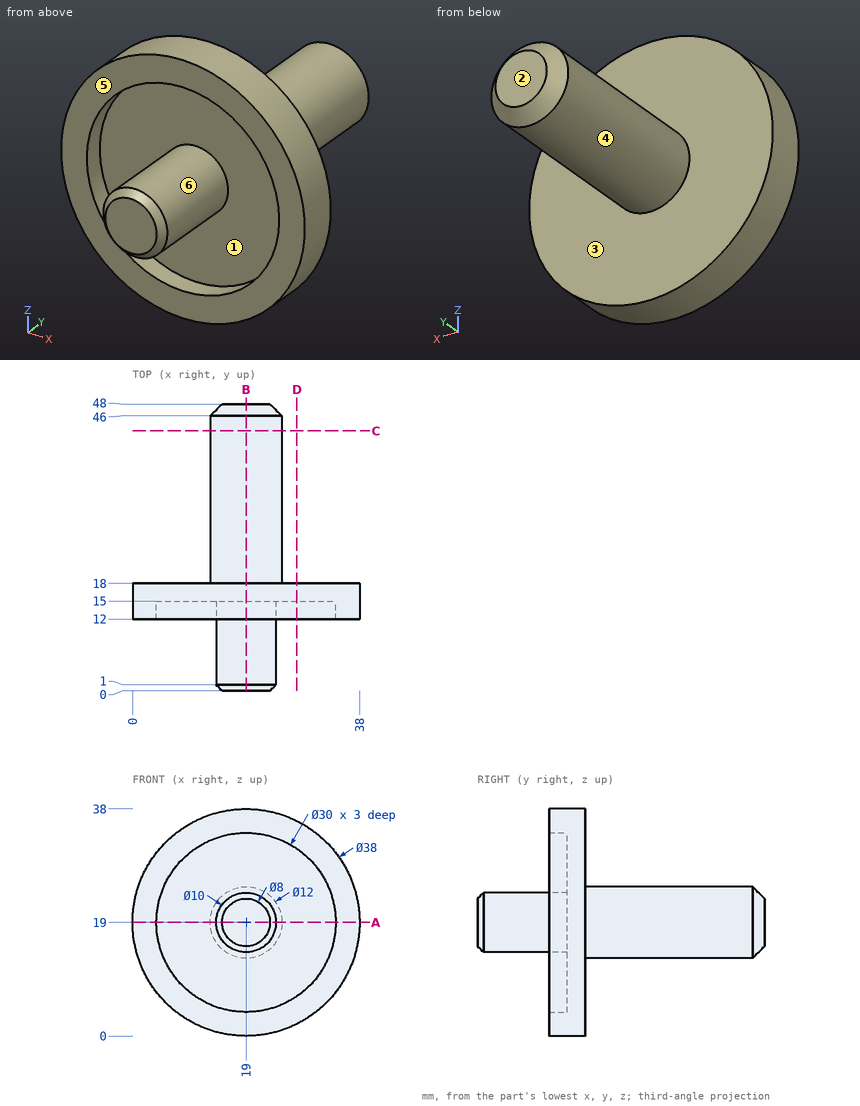
Study the drawing (mm; zero at the part's minimum x, y, z) and answer. A direction names the side the tool comes from. Round coordinates to 2 decimals unless told otherwise and drop trailing zeros. Write each loop counter-clockwise with the first axis right and the second up, starting at its lowest first coordinate (ties: lowest second). Pieces come first, ordered by that corner, then holes. Notation, with made-up numbers: (64, -32) -> (82, -32) arc R12 ccw to (82, -24) -> close; hole circle Ø4 at (58.5, 41.25). An arc over 180 degrees is marked (long way). Use CSV: the item, a comma, the result in double quotes. Start each with the question number.
(1) Section D-D on x = 27.5 is taken. Give the vertices of the cut face in (y, z), then the cut area to 3 significant figures.
(2) Consider L1, parallel to X at y = 13.5, z = 19; L2, parallel to Y at x = 4.5, z = 31; L3, parallel to Y at x = 11.5, z = 20. Determine where each line is inside the solid, lowest interval first. Write a range as from..to.
(3) Section A-A on z = 19 is taken. Give the vertices of the cut face in (x, y).
(4) Section B-B on x = 19 is taken. Give the vertices of the cut face in (y, z).
(5) Section C-C on y = 43.5 is taken. Give the vertices of the cut face in (x, z).
(6) Each of these flat-tipped pins is pushed along its axis until it touches: pin 1 (3 mm diameter, centred on x = 11, z = 22, fed in from -Y); pin 2 (1.5 mm diameter, centred on y = 7.5, z = 15, fed in from +X); pin 3 (6 mm diameter, centred on x = 15.5, y = 20.5, fed in from -Z). Where does it stop, or does it pass through?
(7) Which of the six approach directions +Z, -Z, +X, -X, +Y, -Y give full straight-line access (tool end or side, diameter ignored) to the marked faces 1, 2 and 3?
(8) The mould has two halves that part along Z. Classify the marked faces 4, 5 and 6: released by +Z, released by -Z, zero draft, split by the parting line, or undercut.
A:
1,outline,"(12, 2.01) -> (18, 2.01) -> (18, 35.99) -> (12, 35.99) -> (12, 31.36) -> (15, 31.36) -> (15, 6.64) -> (12, 6.64) -> close"
1,area,"130 mm²"
2,L1,"x = 0..4, 14..24, 34..38"
2,L2,"y = 12..18"
2,L3,"y = 15..18"
3,outline,"(0, 12) -> (4, 12) -> (4, 15) -> (14, 15) -> (14, 1) -> (15, 0) -> (23, 0) -> (24, 1) -> (24, 15) -> (34, 15) -> (34, 12) -> (38, 12) -> (38, 18) -> (25, 18) -> (25, 46) -> (23, 48) -> (15, 48) -> (13, 46) -> (13, 18) -> (0, 18) -> close"
4,outline,"(0, 15) -> (1, 14) -> (15, 14) -> (15, 4) -> (12, 4) -> (12, 0) -> (18, 0) -> (18, 13) -> (46, 13) -> (48, 15) -> (48, 23) -> (46, 25) -> (18, 25) -> (18, 38) -> (12, 38) -> (12, 34) -> (15, 34) -> (15, 24) -> (1, 24) -> (0, 23) -> close"
5,outline,"circle Ø12 at (19, 19)"
6,pin 1,"stops at y = 15"
6,pin 2,"stops at x = 22.8"
6,pin 3,"stops at z = 0.09"
7,face 1,"-Y"
7,face 2,"+Z, -Z, +X, -X, +Y"
7,face 3,"+Y"
8,face 4,"split by the parting line"
8,face 5,"zero draft"
8,face 6,"undercut"
